For this review, take the finished solid that the model builds, in its own axes (mm). Face numbers are marked on the shaded views. Give positions to 0.01 mm unless a question says otherwise; leave off trailing zeros. Write each loop counter-clockwise with the first axis right and the second up, starting at its lowest first coordinate (ties: lowest second). Pieces come first, ordered by that corner, then holes.
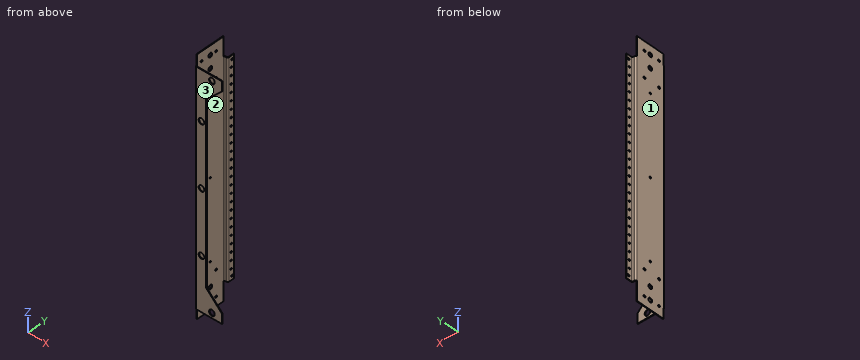
from build123d import *

# Parameters (mm, degrees)
SM_BASE_FLANGE_1_DEPTH     = 394
SKETCH_6_W                 = 13
SKETCH_6_H                 = 60
CUT_EXTRUDE_1_DEPTH        = 24
CUT_EXTRUDE_START          = -4
SKETCH_7_W                 = 81
SKETCH_7_H                 = 33
SKETCH_7_W_2               = 4
CUT_EXTRUDE_2_DEPTH        = 4
SKETCH_8_R                 = 6.5
SKETCH_8_R_2               = 3.25
SKETCH_8_R_3               = 2.5
CUT_EXTRUDE_3_DEPTH        = 10
SKETCH_9_R                 = 3.25
CUT_EXTRUDE_4_DEPTH        = 10
SKETCH_10_R                = 9
CUT_EXTRUDE_5_DEPTH        = 10
SKETCH_11_R                = 2.5
CUT_EXTRUDE_6_DEPTH        = 10
PATTERN_LINEAR_1_COUNT     = 13
PATTERN_LINEAR_1_PITCH     = 25
PATTERN_LINEAR_1_COL_COUNT = 13
PATTERN_LINEAR_1_COL_PITCH = 25
MOVE_START                 = -120
MOVE_BODY_1_DEPTH          = 2
MOVE_BODY_1_2_DEPTH        = 2


# Read off the part's stored shape, not the designer's step: Тело-Переместить/Копировать1
# Sheet-metal steps are written as plain solids
with BuildPart() as part:
    # Sketch 1 → Базовая кромка1 (new, symmetric)
    with BuildSketch(Plane.XY):
        with BuildLine():
            Line((0, 0), (0, -18))
            ThreePointArc((0, -18), (-1.171572875, -20.828427125), (-4, -22))
            Line((-4, -22), (-9, -22))
            ThreePointArc((-9, -22), (-10.414213562, -22.585786438), (-11, -24))
            Line((-11, -24), (-11, -116))
            ThreePointArc((-11, -116), (-10.414213562, -117.414213562), (-9, -118))
            Line((-9, -118), (72, -118))
            Line((72, -118), (72, -120))
            Line((72, -120), (-9, -120))
            ThreePointArc((-9, -120), (-11.828427125, -118.828427125), (-13, -116))
            Line((-13, -116), (-13, -24))
            ThreePointArc((-13, -24), (-11.828427125, -21.171572875), (-9, -20))
            Line((-9, -20), (-4, -20))
            ThreePointArc((-4, -20), (-2.585786438, -19.414213562), (-2, -18))
            Line((-2, -18), (-2, 0))
            Line((-2, 0), (0, 0))
        make_face()
    extrude(amount=SM_BASE_FLANGE_1_DEPTH, both=True)

    # Эскиз6 → Вырез-Вытянуть1 (cut)
    with BuildSketch(Plane(origin=(0, 0, 0), x_dir=(1, 0, 0), z_dir=(0, 1, 0))):
        with Locations((-6.5, -364)):
            Rectangle(SKETCH_6_W, SKETCH_6_H)
        with Locations((-6.5, 364)):
            Rectangle(SKETCH_6_W, SKETCH_6_H)
    extrude(amount=-CUT_EXTRUDE_1_DEPTH, mode=Mode.SUBTRACT)

    # Эскиз7 → Вырез-Вытянуть2 (cut)
    with BuildSketch(Plane.XZ.offset(120).offset(CUT_EXTRUDE_START)):
        with Locations((31.5, -377.5)):
            Rectangle(SKETCH_7_W, SKETCH_7_H)
        Polygon((22, -281), (72, -331), (72, 331), (22, 281), align=None)
        with Locations((31.5, 377.5)):
            Rectangle(SKETCH_7_W, SKETCH_7_H)
        with Locations((-11, -377.5)):
            Rectangle(SKETCH_7_W_2, SKETCH_7_H)
        with Locations((-11, 377.5)):
            Rectangle(SKETCH_7_W_2, SKETCH_7_H)
    extrude(amount=CUT_EXTRUDE_2_DEPTH, mode=Mode.SUBTRACT)

    # Эскиз8 → Вырез-Вытянуть3 (cut)
    with BuildSketch(Plane.ZY.offset(13)):
        with Locations(Location((-365, -70, 0), (0, 0, 270))):
            Circle(SKETCH_8_R)
        with Locations(Location((-325, -70, 0), (0, 0, 270))):
            Circle(SKETCH_8_R)
        with Locations(Location((-365, -50, 0), (0, 0, 270))):
            Circle(SKETCH_8_R_2)
        with Locations(Location((-365, -100, 0), (0, 0, 270))):
            Circle(SKETCH_8_R_2)
        with Locations(Location((-285, -50, 0), (0, 0, 270))):
            Circle(SKETCH_8_R_2)
        with Locations(Location((-285, -100, 0), (0, 0, 270))):
            Circle(SKETCH_8_R_2)
        with Locations(Location((285, -100, 0), (0, 0, 90))):
            Circle(SKETCH_8_R_2)
        with Locations(Location((285, -50, 0), (0, 0, 90))):
            Circle(SKETCH_8_R_2)
        with Locations(Location((365, -100, 0), (0, 0, 90))):
            Circle(SKETCH_8_R_2)
        with Locations(Location((365, -50, 0), (0, 0, 90))):
            Circle(SKETCH_8_R_2)
        with Locations(Location((325, -70, 0), (0, 0, 90))):
            Circle(SKETCH_8_R)
        with Locations(Location((365, -70, 0), (0, 0, 90))):
            Circle(SKETCH_8_R)
        with Locations(Location((-250, -70, 0), (0, 0, 270))):
            Circle(SKETCH_8_R_3)
        with Locations(Location((0, -70, 0), (0, 0, 270))):
            Circle(SKETCH_8_R_3)
        with Locations(Location((250, -70, 0), (0, 0, 270))):
            Circle(SKETCH_8_R_3)
    extrude(amount=-CUT_EXTRUDE_3_DEPTH, mode=Mode.SUBTRACT)

    # Эскиз9 → Вырез-Вытянуть4 (cut)
    with BuildSketch(Plane.ZY.offset(2)):
        with Locations(Location((-322, -7, 0), (0, 0, 270))):
            Circle(SKETCH_9_R)
        with Locations(Location((322, -7, 0), (0, 0, 90))):
            Circle(SKETCH_9_R)
    extrude(amount=-CUT_EXTRUDE_4_DEPTH, mode=Mode.SUBTRACT)

    # Эскиз10 → Вырез-Вытянуть5 (cut)
    with BuildSketch(Plane.XZ.offset(120)):
        with Locations(Location((40, -345, 0), (0, 0, 270))):
            Circle(SKETCH_10_R)
        with Locations(Location((40, 345, 0), (0, 0, 270))):
            Circle(SKETCH_10_R)
        with Locations(Location((7, -7, 0), (0, 0, 270))):
            Circle(SKETCH_10_R)
        with Locations(Location((7, 193, 0), (0, 0, 270))):
            Circle(SKETCH_10_R)
        with Locations(Location((7, -207, 0), (0, 0, 270))):
            Circle(SKETCH_10_R)
    extrude(amount=-CUT_EXTRUDE_5_DEPTH, mode=Mode.SUBTRACT)

    # Эскиз11 → Вырез-Вытянуть6 (cut)
    with BuildSketch(Plane.ZY.offset(2)):
        with Locations(Location((0, -10, 0), (0, 0, 270))):
            Circle(SKETCH_11_R)
    cut_extrude_6 = extrude(amount=-CUT_EXTRUDE_6_DEPTH, mode=Mode.SUBTRACT)

    # Линейный массив1: Вырез-Вытянуть6 ×13
    with Locations(*[(0, 0, i * PATTERN_LINEAR_1_PITCH) for i in range(1, PATTERN_LINEAR_1_COUNT)]):
        add(cut_extrude_6, mode=Mode.SUBTRACT)

    # Линейный массив1 col: Вырез-Вытянуть6 ×13
    with Locations(*[(0, 0, -i * PATTERN_LINEAR_1_COL_PITCH) for i in range(1, PATTERN_LINEAR_1_COL_COUNT)]):
        add(cut_extrude_6, mode=Mode.SUBTRACT)

    # Move Body 1 outline → Move Body 1 (cut)
    with BuildSketch(Plane(origin=(0, 0, 0), x_dir=(1, 0, 0), z_dir=(0, 1, 0)).offset(MOVE_START)):
        with BuildLine():
            ThreePointArc((1.343145751, 200), (7, 184), (12.656854249, 200))
            ThreePointArc((12.656854249, 200), (7, 198), (1.343145751, 200))
        make_face()
        with BuildLine():
            ThreePointArc((1.343145751, 0), (7, -16), (12.656854249, 0))
            ThreePointArc((12.656854249, 0), (7, -2), (1.343145751, 0))
        make_face()
        with BuildLine():
            ThreePointArc((1.343145751, -200), (7, -216), (12.656854249, -200))
            ThreePointArc((12.656854249, -200), (7, -202), (1.343145751, -200))
        make_face()
    extrude(amount=MOVE_BODY_1_DEPTH, mode=Mode.SUBTRACT)

    # Move Body 1 2 outline → Move Body 1 2 (add)
    with BuildSketch(Plane(origin=(0, 0, 0), x_dir=(1, 0, 0), z_dir=(0, 1, 0)).offset(MOVE_START)):
        with BuildLine():
            ThreePointArc((1.343145751, 200), (7, 202), (12.656854249, 200))
            ThreePointArc((12.656854249, 200), (7, 216), (1.343145751, 200))
        make_face()
        with BuildLine():
            ThreePointArc((1.343145751, 0), (7, 2), (12.656854249, 0))
            ThreePointArc((12.656854249, 0), (7, 16), (1.343145751, 0))
        make_face()
        with BuildLine():
            ThreePointArc((1.343145751, -200), (7, -198), (12.656854249, -200))
            ThreePointArc((12.656854249, -200), (7, -184), (1.343145751, -200))
        make_face()
    extrude(amount=MOVE_BODY_1_2_DEPTH)


solid = part.part
(1) The part is to be moulded in two halves that separate along Y. For the marked faces 1, 2 and 3, say which applies: +Y half, -Y half, draft (parallel to the pull), parting line (faces both ways), or undercut.
(2) For L1, parallel to Z at x = -11.7, y = -50; L2, parallel to Y at x = -12, z = -365; L3, parallel to Y at x = -3.5, z = -302, list the stretches that pass through material, from the lowest coordinate up.
(3) We need section B-B (z = 88). Write out the cut boundary in (x, y).
(4) Clearance check with flat-ended pins moving along their axes: pin 1 Ø1.5 at (x, z) = (13.5, 119) entering from +Y; pin 2 Ø6 at (y, z) = (-10, -25) entering from +X; pin 3 Ø17 at (y, z) = (-70, -365) entering from +X; pin 4 Ø3 at (y, z) = (-10, 200) entering from +X. State where each tip first meets the part, or that it passes through.
(5) We need section A-A (x = 40). Write out the cut boundary in (y, z), and give its area (3 significant figures).
The answers:
1. face 1: draft
1. face 2: undercut
1. face 3: -Y half
2. L1: z = -394 to -368.25, -361.75 to -288.25, -281.75 to 281.75, 288.25 to 361.75, 368.25 to 394
2. L2: y = -116 to -103.25, -96.75 to -76.5, -63.5 to -53.25, -46.75 to -24
2. L3: y = -120 to -118, -21.97 to -19.94
3. outline: (-13, -116) arc R4 ccw to (-9, -120) - (22, -120) - (22, -118) - (-9, -118) arc R2 cw to (-11, -116) - (-11, -24) arc R2 cw to (-9, -22) - (-4, -22) arc R4 ccw to (0, -18) - (0, 0) - (-2, 0) - (-2, -18) arc R2 cw to (-4, -20) - (-9, -20) arc R4 ccw to (-13, -24) - close
4. pin 1: stops at y = -118
4. pin 2: stops at x = 0
4. pin 3: stops at x = -11
4. pin 4: passes through
5. outline: (-120, -361) - (-118, -361) - (-118, -354) - (-120, -354) - close; (-120, -336) - (-118, -336) - (-118, -299) - (-120, -299) - close; (-120, 299) - (-118, 299) - (-118, 336) - (-120, 336) - close; (-120, 354) - (-118, 354) - (-118, 361) - (-120, 361) - close
5. area: 176 mm2
